Build history of the part. All positions in model axes, mm. Coordinates: 2 decimals unless noted, no trailing zeros. Order: outer loops, then holes, each group sorted by start corner. A loop starts at its lowest first (then second) coordinate and runs counter-clockwise, first axis right, second up. Notation, with made-up numbers: M -18.5,64 L -12.5,64 A17 ccw -12.5,75 Z; hole C 4,81 d8. An arc over 180 degrees is marked long. Write item = value, one per line. Start each with the question number.
Q1. Band-saw the part on A-A on z = -5. Write the cut outline in (x, y) (3 decimals), plus the area to 3 significant figures.
Q2. Pin check, flat tip, straight feed: P1, Ø1.5, axis at x = -4.5, y = 26.5, coming from the +Z side. Stop position of the tip, or through.
Q3. Drill centre lines: probe 1 along Z at (x, y) = (-15, -139); probe 2 along X at (y, z) = (279.5, -6.5) (3 decimals); probe 3 along Z at (x, y) = (-9, -134) (3 decimals). Where is each one in solid material? Low to high.
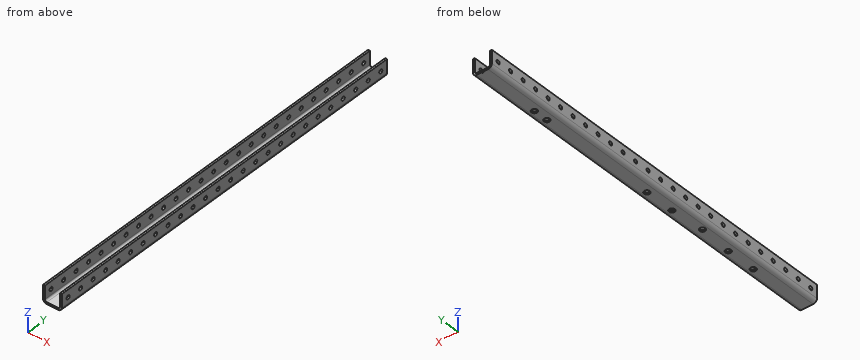
```python
from build123d import *

# Parameters (mm, degrees)
BOSS_EXTRUDE1_DEPTH = 330.2
SKETCH3_R           = 1.651
SKETCH3_R_2         = 4.826
CUT_EXTRUDE1_DEPTH  = 332.814083863
SKETCH4_R           = 3.175
CUT_EXTRUDE2_DEPTH  = 333.951397542
LPATTERN1_COUNT     = 26
LPATTERN1_PITCH     = 25.4


with BuildPart() as part:
    # Sketch2 → Boss-Extrude1 (new, symmetric)
    with BuildSketch(Plane(origin=(0, 0, 0), x_dir=(1, 0, 0), z_dir=(0, 1, 0))):
        with BuildLine():
            Line((-12.7, 0), (-12.7, 22.225))
            ThreePointArc((-12.7, 22.225), (-11.77006403, 24.47006403), (-9.525, 25.4))
            Line((-9.525, 25.4), (9.525, 25.4))
            ThreePointArc((9.525, 25.4), (11.77006403, 24.47006403), (12.7, 22.225))
            Line((12.7, 22.225), (12.7, 0))
            Line((12.7, 0), (15.875, 0))
            Line((15.875, 0), (15.875, 22.225))
            ThreePointArc((15.875, 22.225), (14.015128061, 26.715128061), (9.525, 28.575))
            Line((9.525, 28.575), (-9.525, 28.575))
            ThreePointArc((-9.525, 28.575), (-14.015128061, 26.715128061), (-15.875, 22.225))
            Line((-15.875, 22.225), (-15.875, 0))
            Line((-15.875, 0), (-12.7, 0))
        make_face()
    extrude(amount=BOSS_EXTRUDE1_DEPTH, both=True)

    # Sketch3 → Cut-Extrude1 (cut, through all)
    with BuildSketch(Plane(origin=(0, 0, -28.575), x_dir=(-1, 0, 0), z_dir=(0, 0, -1))):
        with Locations((0, 330.2)):
            Circle(SKETCH3_R)
        with Locations((-2.032, 222.25)):
            Circle(SKETCH3_R_2)
        with Locations((-2.032, 196.85)):
            Circle(SKETCH3_R_2)
        with Locations((-2.032, -6.35)):
            Circle(SKETCH3_R_2)
        with Locations((-2.032, -57.15)):
            Circle(SKETCH3_R_2)
        with Locations((2.032, -114.3)):
            Circle(SKETCH3_R_2)
        with Locations((-2.032, -171.45)):
            Circle(SKETCH3_R_2)
        with Locations((-2.032, -222.25)):
            Circle(SKETCH3_R_2)
    extrude(amount=-CUT_EXTRUDE1_DEPTH, mode=Mode.SUBTRACT)

    # Sketch4 → Cut-Extrude2 (cut, through all)
    with BuildSketch(Plane(origin=(15.875, 0, 0), x_dir=(0, 0, -1), z_dir=(1, 0, 0))):
        with Locations((12.7, 317.5)):
            Circle(SKETCH4_R)
    cut_extrude2 = extrude(amount=-CUT_EXTRUDE2_DEPTH, mode=Mode.SUBTRACT)

    # LPattern1: Cut-Extrude2 ×26
    with Locations(*[(0, -i * LPATTERN1_PITCH, 0) for i in range(1, LPATTERN1_COUNT)]):
        add(cut_extrude2, mode=Mode.SUBTRACT)


solid = part.part
```
Recorded:
q1.outline = M -15.875,-330.2 L -12.7,-330.2 L -12.7,330.2 L -15.875,330.2 Z; M 12.7,-330.2 L 15.875,-330.2 L 15.875,330.2 L 12.7,330.2 Z
q1.area = 4,190 mm2
q2.P1 = -25.4
q3.probe_1 = -25.44 to -15.8, -9.6 to 0
q3.probe_2 = -15.875 to -12.7, 12.7 to 15.875
q3.probe_3 = -28.575 to -25.4
